Answer from the drawing. Dimensions are ordinates in mm from the lowest x, y and z of the part. A direction names the side the tool comes from. Round coordinates to 2 decimals unless told otherwise and drop trailing zeros. Loops run counter-clockwise (first coordinate to the right, second up) from the corner with the lowest first, then second, coordinate; pieces in that order, holes last. Notation, with made-up numbers: M -9.75,32 L 21.25,32 A27 ccw 21.25,52 Z; hole C 0,-18.75 d1. An arc over 180 degrees is marked long. Answer as a JSON object with one key per item and string values.
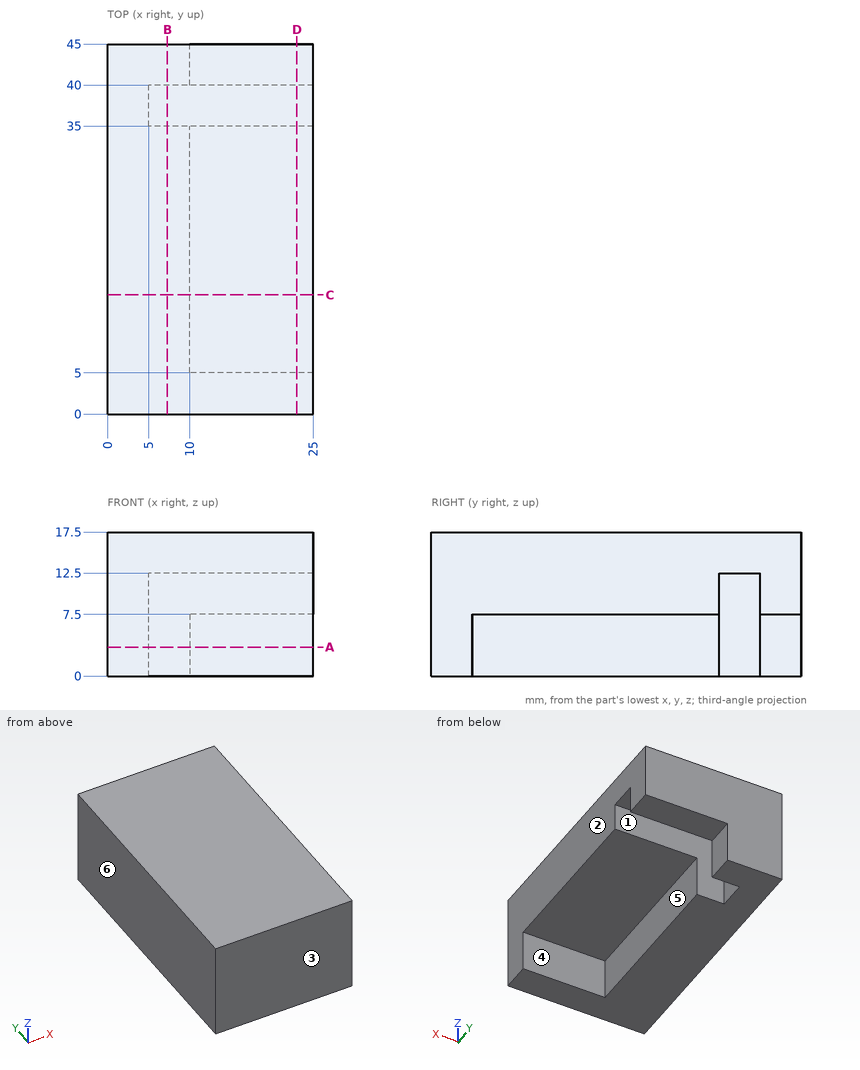
Item 1: The part is cut by section B-B (x = 7.25). Give the vertices of the cut face in (y, z).
Values follow:
{"outline": "M 0,0 L 35,0 L 35,12.5 L 40,12.5 L 40,0 L 45,0 L 45,17.5 L 0,17.5 Z"}
Item 2: Straight lines are drawn through the part: line 1 (Y direction, x = 17.5, z = 8.75); line 2 (Z direction, x = 19.5, y = 18); line 3 (X direction, y = 16.5, z = 6.5). For each, find the intervals that lie inside material, in ascending order.
Values follow:
{"line 1": "0 to 35, 40 to 45", "line 2": "7.5 to 17.5", "line 3": "0 to 10"}
Item 3: The part is cut by section A-A (z = 3.5). Give the vertices of the cut face in (x, y).
Values follow:
{"outline": "M 0,0 L 25,0 L 25,5 L 10,5 L 10,35 L 5,35 L 5,40 L 10,40 L 10,45 L 0,45 Z"}
Item 4: The part is cut by section D-D (x = 23). Give the vertices of the cut face in (y, z), then the cut area to 4 significant figures.
Values follow:
{"outline": "M 0,0 L 5,0 L 5,7.5 L 35,7.5 L 35,12.5 L 40,12.5 L 40,7.5 L 45,7.5 L 45,17.5 L 0,17.5 Z", "area": "462.5 mm^2"}
Item 5: The part is cut by section C-C (y = 14.5). Give the vertices of the cut face in (x, z).
Values follow:
{"outline": "M 0,0 L 10,0 L 10,7.5 L 25,7.5 L 25,17.5 L 0,17.5 Z"}
Item 6: Which of the six approach directions +Z, -Z, +X, -X, +Y, -Y give full straight-line access (tool end or side, diameter ignored) to the marked faces 5 and 6?
Values follow:
{"face 5": "-Z, +X, +Y", "face 6": "+Z, -Z, -X, +Y, -Y"}
Item 7: Flat-ended cylindrical pins translate along their axes: P1, Ø2.5, axis at y = 41.5, z = 5, coming from the +X side; P2, Ø6, axis at x = 15.5, z = 7, coming from the -Y side; P3, Ø1.5, axis at y = 38, z = 4.5, coming from the +X side; P4, Ø2.5, axis at x = 16, y = 37, coming from the -Z side. Find the tip coordinate at first contact, or state that the pin passes through.
Values follow:
{"P1": "x = 10", "P2": "y = 0", "P3": "x = 5", "P4": "z = 12.5"}
Item 8: Determine the mould class of the marked faces 1, 2, 3 and 4 for opening direction Y: released by +Y, released by -Y, zero draft, split by the parting line, or undercut.
Values follow:
{"face 1": "undercut", "face 2": "zero draft", "face 3": "released by -Y", "face 4": "released by +Y"}
